Read the model definition and answer for the solid it produces. Units are mm, in the model's axes. A direction names the side the tool comes from. Coordinates: 2 decimals unless noted, no trailing zeros. Write each loop counter-clockwise with the first axis right and the second up, starting at its lowest first coordinate (ties: lowest second). Pieces come first, ordered by that corner, then holes.
Item 1: Section C-C (y = 148) is taken. Give the vertices of the cut face in (x, z), then the cut area to 3 significant figures.
Item 2: Determine the mould class of faces 1 (the face through (-258, 150, 150)), 2 (the face through (-258, -88, -175)), 3 (the face through (-257.721, 43.483, 150.318)) for opening direction Y: released by +Y, released by -Y, zero draft, split by the parting line, or undercut.
Item 3: Section B-B (x = -282.5) is taken. Give the vertices of the cut face in (y, z), then the cut area to 3 significant figures.
Item 4: A tool of negligible diameter and unlimited length cuts with its end or side. For faces 4 (the face through (-258, -25, 65)), 5 (the face through (-258, 175, -2)), from which of +Z, -Z, +X, -X, +Y, -Y can it reach the whole face along a straight path? Write none if from no direction.
Item 5: Straight lines are drawn through the part: probe 1 along Y at (x, z) = (-46, 40.5); probe 2 along Y at (x, z) = (-215, 157.5); probe 3 along Z at (x, y) = (-421, -16). For each, find the intervals that lie inside material, in ascending order.
Item 6: Each of these flat-tipped pins is pushed along its axis until it touches: P1, Ø2, axis at x = -244, y = 11, coming from the +Z side; P2, Ø2, axis at x = -315, y = 1.5, coming from the +Z side; P3, Ø4, axis at x = -138.5, y = -138, coming from the +Z side. Where does it stop, or does it pass through?
Item 7: Section A-A (z = 28) is taken. Give the vertices of the cut face in (x, y), then the cut area to 3 significant figures.
from build123d import *


with BuildPart() as f2:
    # F2: sweep along a path in F1
    with BuildLine(Plane.XZ) as f2_path:
        Line((0, 0), (-508.3263516426, 0))
    # F0 (on Right) → F2 (sweep)
    with BuildSketch(Plane.YZ):
        with BuildLine():
            Line((175, 125), (125, 175))
            Line((125, 175), (50, 175))
            ThreePointArc((50, 175), (43.3012701892, 150), (25, 131.6987298108))
            Line((25, 131.6987298108), (25, 0))
            Line((25, 0), (25, -131.6987298108))
            ThreePointArc((25, -131.6987298108), (43.3012701892, -150), (50, -175))
            Line((50, -175), (125, -175))
            Line((125, -175), (175, -125))
            Line((175, -125), (175, 125))
        make_face()
        with BuildLine():
            Line((25, -131.6987298108), (25, 0))
            ThreePointArc((25, 0), (17.6776695297, -17.6776695297), (0, -25))
            ThreePointArc((0, -25), (-17.6776695297, -17.6776695297), (-25, 0))
            Line((-25, 0), (-25, -131.6987298108))
            ThreePointArc((-25, -131.6987298108), (0, -125), (25, -131.6987298108))
        make_face()
        with BuildLine():
            Line((-25, 0), (-25, 131.6987298108))
            ThreePointArc((-25, 131.6987298108), (-43.3012701892, 150), (-50, 175))
            Line((-50, 175), (-125, 175))
            Line((-125, 175), (-175, 125))
            Line((-175, 125), (-175, -125))
            Line((-175, -125), (-125, -175))
            Line((-125, -175), (-50, -175))
            ThreePointArc((-50, -175), (-43.3012701892, -150), (-25, -131.6987298108))
            Line((-25, -131.6987298108), (-25, 0))
        make_face()
    sweep(path=f2_path.line)


solid = f2.part
Established:
1. outline: (-508.33, -152) - (0, -152) - (0, 152) - (-508.33, 152) - close
1. area: 155,000 mm2
2. face 1: released by +Y
2. face 2: zero draft
2. face 3: undercut
3. outline: (-175, -125) - (-125, -175) - (-50, -175) arc R50 cw to (50, -175) - (125, -175) - (175, -125) - (175, 125) - (125, 175) - (50, 175) arc R50 cw to (25, 131.7) - (25, 0) arc R25 cw to (-25, 0) - (-25, 131.7) arc R50 cw to (-50, 175) - (-125, 175) - (-175, 125) - close
3. area: 102,000 mm2
4. face 4: +Z, +X, -X
4. face 5: +Z, -Z, +X, -X, +Y
5. probe 1: y = -175 to -25, 25 to 175
5. probe 2: y = -142.5 to -46.84, 46.84 to 142.5
5. probe 3: z = -127.63 to -19.21
6. P1: stops at z = -21.93
6. P2: stops at z = -24.87
6. P3: stops at z = 164
7. outline: (-508.33, -175) - (0, -175) - (0, -25) - (-508.33, -25) - close; (-508.33, 25) - (0, 25) - (0, 175) - (-508.33, 175) - close
7. area: 152,000 mm2
